```python
from build123d import *

# Parameters (mm, degrees)
ESQUISSE1_W                = 550
ESQUISSE1_H                = 1250
ESQUISSE1_W_2              = 125
ESQUISSE1_H_2              = 525
ESQUISSE1_W_3              = 200
ESQUISSE1_W_4              = 400
ESQUISSE1_H_3              = 500
BOSS_EXTRU_1_DEPTH         = 63
R_P_TITION_LIN_AIRE1_COUNT = 2
R_P_TITION_LIN_AIRE1_PITCH = 263
ESQUISSE2_W                = 75
ESQUISSE2_H                = 75
ESQUISSE2_W_2              = 74.718169062
BOSS_EXTRU_2_DEPTH         = 200
BOSS_EXTRU_4_DEPTH         = 550
BOSS_EXTRU_4_DEPTH_BACK    = 550
ESQUISSE7_W                = 63
ESQUISSE7_H                = 75
ESQUISSE3_R                = 10
ENL_V_MAT_EXTRU_2_DEPTH    = 1513.921759378
BOSS_EXTRU_5_DEPTH         = 63
BOSS_EXTRU_6_DEPTH         = 5
ESQUISSE12_R               = 7.355365699
ENL_V_MAT_EXTRU_3_DEPTH    = 100
R_P_TITION_LIN_AIRE2_COUNT = 12
R_P_TITION_LIN_AIRE2_PITCH = 50
BOSS_EXTRU_7_START         = -263
ESQUISSE13_R               = 9.503964929
BOSS_EXTRU_7_DEPTH         = 200


with BuildPart() as part:
    # Esquisse1 → Boss.-Extru.1 (new body)
    with BuildSketch(Plane.XY):
        with Locations((275, 625)):
            Rectangle(ESQUISSE1_W, ESQUISSE1_H)
        with Locations((137.5, 337.5)):
            Rectangle(ESQUISSE1_W_2, ESQUISSE1_H_2, mode=Mode.SUBTRACT)
        with Locations((375, 337.5)):
            Rectangle(ESQUISSE1_W_3, ESQUISSE1_H_2, mode=Mode.SUBTRACT)
        with Locations((275, 925)):
            Rectangle(ESQUISSE1_W_4, ESQUISSE1_H_3, mode=Mode.SUBTRACT)
    extrude(amount=BOSS_EXTRU_1_DEPTH)


with BuildPart() as r_p_tition_lin_aire1_1:
    # R_p_tition lin_aire1: pattern copy
    add(part.part.moved(Location(Vector(0, 0, 1) * (1 * R_P_TITION_LIN_AIRE1_PITCH))))


with BuildPart() as part_1:
    add(part.part)

    add(r_p_tition_lin_aire1_1.part)  # Boss.-Extru.2 merges R_p_tition lin_aire1_1
    # Esquisse2 → Boss.-Extru.2 (add)
    with BuildSketch(Plane.XY.offset(63)):
        with Locations((37.5, 37.5)):
            Rectangle(ESQUISSE2_W, ESQUISSE2_H)
        with Locations((512.359084531, 37.5)):
            Rectangle(ESQUISSE2_W_2, ESQUISSE2_H)
        with Locations((512.359084531, 1212.5)):
            Rectangle(ESQUISSE2_W_2, ESQUISSE2_H)
        with Locations((37.5, 1212.5)):
            Rectangle(ESQUISSE2_W, ESQUISSE2_H)
    extrude(amount=BOSS_EXTRU_2_DEPTH)


with BuildPart() as body_2:
    # Esquisse7 → Boss.-Extru.4 (new, two sides: drawn at the far end of the back side and taken through both)
    with BuildSketch(Plane.ZY.offset(-237.5).offset(-BOSS_EXTRU_4_DEPTH_BACK)):
        with Locations((167.0850662, 639.649163537)):
            Rectangle(ESQUISSE7_W, ESQUISSE7_H)
    extrude(amount=BOSS_EXTRU_4_DEPTH + BOSS_EXTRU_4_DEPTH_BACK)


with BuildPart() as enl_v_mat_extru_2_tool:
    # Esquisse3 → Enl_v. mat.-Extru.2 (new, through all)
    with BuildSketch(Plane.XY.offset(326)):
        with Locations((237.5, 637.5)):
            Circle(ESQUISSE3_R)
    extrude(amount=-ENL_V_MAT_EXTRU_2_DEPTH)


with BuildPart() as part_2:
    add(part_1.part)

    # Enl_v. mat.-Extru.2: cut by enl_v_mat_extru_2_tool
    add(enl_v_mat_extru_2_tool.part, mode=Mode.SUBTRACT)



with BuildPart() as body_2_1:
    add(body_2.part)

    # Enl_v. mat.-Extru.2: cut by enl_v_mat_extru_2_tool
    add(enl_v_mat_extru_2_tool.part, mode=Mode.SUBTRACT)



with BuildPart() as body_3:
    # Esquisse11 → Boss.-Extru.5 (new body)
    with BuildSketch(Plane.XY.offset(198.5850662)):
        with BuildLine():
            Line((-99.153084709, 586.914270743), (330.503621206, 226.557033524))
            Line((330.503621206, 226.557033524), (284.435304351, 171.629424966))
            Line((284.435304351, 171.629424966), (-145.221401564, 531.986662185))
            ThreePointArc((-145.221401564, 531.986662185), (-149.651047416, 582.484624891), (-99.153084709, 586.914270743))
        make_face()
    extrude(amount=-BOSS_EXTRU_5_DEPTH)


with BuildPart() as body_2_2:
    add(body_2_1.part)

    add(body_3.part)  # Boss.-Extru.6 merges body 3
    # Esquisse11_3 → Boss.-Extru.6 (add)
    with BuildSketch(Plane.XY.offset(198.5850662)):
        with BuildLine():
            Line((-114.54998443, 559.450466464), (-114.54998443, 643.613737641))
            ThreePointArc((-114.54998443, 643.613737641), (-123.445013511, 652.508766722), (-132.340042592, 643.613737641))
            Line((-132.340042592, 643.613737641), (-132.340042592, 559.450466464))
            ThreePointArc((-132.340042592, 559.450466464), (-123.445013511, 550.555437383), (-114.54998443, 559.450466464))
        make_face()
    extrude(amount=BOSS_EXTRU_6_DEPTH)

    # Esquisse12 → Enl_v. mat.-Extru.3 (cut)
    with BuildSketch(Plane.XY.offset(198.5850662)):
        with Locations((-123.445013511, 559.450466464)):
            Circle(ESQUISSE12_R)
    enl_v_mat_extru_3 = extrude(amount=-ENL_V_MAT_EXTRU_3_DEPTH, mode=Mode.SUBTRACT)

    # R_p_tition lin_aire2: Enl_v. mat.-Extru.3 ×12
    with Locations(*[Vector(0.7661915431257939, -0.6426122619764696, 0) * (i * R_P_TITION_LIN_AIRE2_PITCH) for i in range(1, R_P_TITION_LIN_AIRE2_COUNT)]):
        add(enl_v_mat_extru_3, mode=Mode.SUBTRACT)


with BuildPart() as part_3:
    add(part_2.part)

    add(body_2_2.part)  # Boss.-Extru.7 merges body 2
    # Esquisse13 → Boss.-Extru.7 (add)
    with BuildSketch(Plane.XY.offset(326).offset(BOSS_EXTRU_7_START)):
        with Locations((237.5, 257.608372702)):
            Circle(ESQUISSE13_R)
    extrude(amount=BOSS_EXTRU_7_DEPTH)


solid = part_3.part
```
Source: CAD feature listing. Evaluate the final solid. Frame: model axes, mm. A direction names the side the tool comes from. Round coordinates to 2 decimals unless told otherwise and drop trailing zeros. Loops run counter-clockwise (first coordinate to the right, second up) from the corner with the lowest first, then second, coordinate; pieces in that order, holes last.
1. Contact query for flat-ended pins moving along their axis: pin 1 (6 mm diameter, centred on x = 187.5, z = 146, fed in from -Y); pin 2 (6.5 mm diameter, centred on x = -121.5, y = 597, fed in from -Z); pin 3 (19 mm diameter, centred on x = -85.14, y = 527.32, fed in from +Z). Output: stop coordinate, or through.
2. Section query A-A on y = 777.5. Output: boundary loops of the cut face in (x, z), and give its area (3 significant figures).
3. Ray query, L1, parallel to X at y = 567.5, z = 50.5; L2, parallel to X at y = 637, z = 301; L3, parallel to Y at x = -119, z = 192. Return the intervals inside material, ascending.
4. Mould query, pull axis X, two halves, no side actions, for faces 1 (the flat face through (37, 75, 162)), 2 (the flat face through (72.6, 349.3, 167.5)), 3 (the flat face through (75, 334, 294)), 4 (the flat face through (272, 675, 294)). Classes: released by +X, released by -X, zero draft, split by the parting line, or undercut.
5. Access query for faces 5 (the flat face through (112.668, 409.258, 167.526)), 6 (the flat face through (512, 1175, 162)), 7 (the flat face through (75, 922, 31)). Directions: +Z, -Z, +X, -X, +Y, -Y. A direction counts if a zero-diameter tool reaches every point of the face in a straight line with its end or side. Return the directions, or none.
6. Section query D-D on z = 161. Give the number of separate pieces and of enclosed holes in the cut face, and give its area (3 significant figures).
7. Section query B-B on z = 294.5. Output: boundary loops of the cut face in (x, y), and give its area (3 significant figures).
8. Section query C-C on x = 564.5. Output: boundary loops of the cut face in (y, z).
Answers below:
1. pin 1: stops at y = 250.41
1. pin 2: stops at z = 135.59
1. pin 3: stops at z = 198.59
2. outline: (0, 0) - (75, 0) - (75, 63) - (0, 63) - close; (0, 263) - (75, 263) - (75, 326) - (0, 326) - close; (475, 0) - (550, 0) - (550, 63) - (475, 63) - close; (475, 263) - (550, 263) - (550, 326) - (475, 326) - close
2. area: 18,900 mm2
3. L1: x = 0 to 75, 200 to 275, 475 to 550
3. L2: x = 0 to 227.51, 247.49 to 550
3. L3: y = 509.99 to 553.59, 565.31 to 595.15, 602.15 to 677.15
4. face 1: zero draft
4. face 2: released by -X
4. face 3: undercut
4. face 4: undercut
5. face 5: +X
5. face 6: +X, -X
5. face 7: +Z, -Z
6. separate pieces: 6
6. enclosed holes: 13
6. area: 145,000 mm2
7. outline: (0, 0) - (550, 0) - (550, 1250) - (0, 1250) - close; hole (75, 75) - (200, 75) - (200, 600) - (75, 600) - close; hole (75, 675) - (475, 675) - (475, 1175) - (75, 1175) - close; hole circle Ø20 at (237.5, 637.5); hole (275, 75) - (475, 75) - (475, 600) - (275, 600) - close
7. area: 317,000 mm2
8. outline: (602.15, 135.59) - (677.15, 135.59) - (677.15, 198.59) - (602.15, 198.59) - close
